Autodesk Inventor part; units mm, degrees
ref_plane "YZ Plane" through (0, 0, 0) normal (1, 0, 0) x (0, 1, 0)
ref_plane "XZ Plane" through (0, 0, 0) normal (0, 1, 0) x (-1, 0, 0)
ref_plane "XY Plane" through (0, 0, 0) normal (0, 0, 1) x (1, 0, 0)
sketch "Sketch1" plane through (0, 0, 0) normal (0, 1, 0) x (-1, 0, 0)
  circle A0 centre (0, 0) radius 3
  circle A1 centre (0, 0) radius 2.75
  dimension "d0" = 6
  dimension "d1" = 5.5
extrude "Extrusion1" add sketch "Sketch1" along normal blind 25 contours A0 | A1
chamfer "Chamfer1" distance 0.3 angle 45 2 edges at (3, 25, 0) (3, 0, 0) measured on face at (-2.9612, 8.3333, -0.4812)
sketch "Sketch2" plane through (0, 25, 0) normal (0, 1, 0) x (1, 0, 0)
  circle A0 centre (0, 0) radius 2.5
  dimension "d7" = 5
extrude "Extrusion2" cut sketch "Sketch2" against normal blind 50
properties part number "26-10-211"
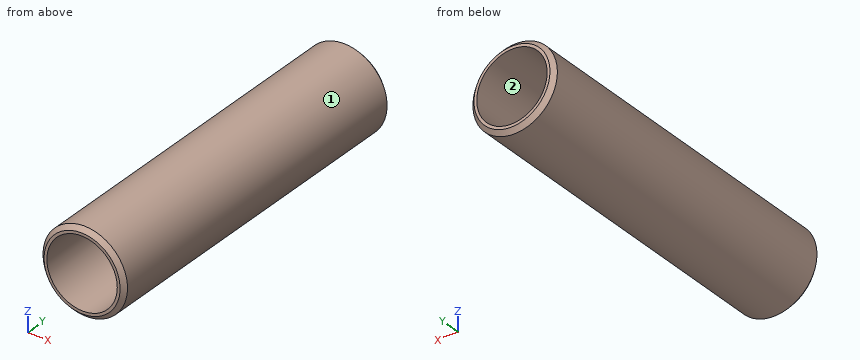
Read the model definition and answer for the solid it produces. Units are mm, in the model's axes. Face numbers are marked on the shaded views. Give positions to 0.01 mm unless a question says otherwise; leave off trailing zeros. Loops run counter-clockwise (first coordinate to the right, second up) from the corner with the lowest first, then second, coordinate; pieces in that order, holes last.
Item 1: The part is cut by section B-B (x = 0). Write down the section's boundary in (y, z).
Item 2: The part is cut by section A-A (z = 0). Write down the section's boundary in (x, y), and give its area (3 significant figures).
Item 3: Find the intervals of material crossed by line 1 along X through (y, z) = (9.25, -0.1); line 2 along X through (y, z) = (9.25, 2.25), in increasing order.
Item 4: Each of these flat-tipped pins is pushed along its axis until it touches: pin 1 Ø1 at (x, y) = (-2, 15) entering from -Z; pin 2 Ø3 at (x, y) = (2, 10) entering from -Z. Where does it stop, or does it pass through?
Item 5: The part is cut by section C-C (y = 10.5). Write down the section's boundary in (x, z), and give its area (3 significant figures).
Item 6: The mould has two halves that part along X. Classify the marked faces 1 and 2: released by +X, released by -X, zero draft, split by the parting line, or undercut.
Taken from the geometry:
1. outline: (0, -2.7) - (0.3, -3) - (24.7, -3) - (25, -2.7) - (25, -2.5) - (0, -2.5) - close; (0, 2.5) - (25, 2.5) - (25, 2.7) - (24.7, 3) - (0.3, 3) - (0, 2.7) - close
2. outline: (-3, 0.3) - (-2.7, 0) - (-2.5, 0) - (-2.5, 25) - (-2.7, 25) - (-3, 24.7) - close; (2.5, 0) - (2.7, 0) - (3, 0.3) - (3, 24.7) - (2.7, 25) - (2.5, 25) - close
2. area: 24.8 mm2
3. line 1: x = -3 to -2.5, 2.5 to 3
3. line 2: x = -1.98 to -1.09, 1.09 to 1.98
4. pin 1: stops at z = -2.6
4. pin 2: stops at z = -2.96
5. outline: circle Ø6 at (0, 0); hole circle Ø5 at (0, 0)
5. area: 8.64 mm2
6. face 1: split by the parting line
6. face 2: undercut
